Design review of the part built by this model. Coordinates are the model's own, in mm. A direction names the side the tool comes from. Coordinates: 2 decimals unless noted, no trailing zeros. Loops run counter-clockwise (first coordinate to the right, second up) from the corner with the lowest first, then second, coordinate; pieces in that order, holes last. Notation, with made-up numbers: (73, -8.5) - (104, -8.5) arc R20 ccw to (104, 0.5) - close; hole circle Ø4 at (58, -33.75). An arc over 180 degrees is marked (long way). One line per question, with ' | ' between items.
from build123d import *

# Parameters (mm, degrees)
SKETCH1_W           = 12.7
SKETCH1_H           = 12.7
BOSS_EXTRUDE1_DEPTH = 2.54
FILLET1_R           = 0.635
SHELL1_START        = 0.635
SHELL1_OUTLINE_W    = 1.905
SHELL1_OUTLINE_H    = 11.43
SHELL1_DEPTH        = 11.43
SKETCH2_R           = 2.54
BOSS_EXTRUDE2_DEPTH = 1.905
BOSS_EXTRUDE3_DEPTH = 0.00254


# Read off the part's stored shape, not the designer's step: Shell1
with BuildPart() as part:
    # Sketch1 → Boss-Extrude1 (new body)
    with BuildSketch(Plane(origin=(0, 0, 0), x_dir=(1, 0, 0), z_dir=(0, 1, 0))):
        with Locations((6.35, 6.35)):
            Rectangle(SKETCH1_W, SKETCH1_H)
    extrude(amount=BOSS_EXTRUDE1_DEPTH)

    # Fillet1
    fillet1_edges = [part.edges().sort_by_distance(p)[0] for p in [
        (0, 1.27, -12.7),
        (12.7, 1.27, -12.7),
        (12.7, 1.27, 0),
        (0, 1.27, 0),
    ]]
    fillet(fillet1_edges, radius=FILLET1_R)

    # Shell1 outline → Shell1 (cut)
    with BuildSketch(Plane.YZ.offset(SHELL1_START)):
        with Locations((0.9525, -6.35)):
            Rectangle(SHELL1_OUTLINE_W, SHELL1_OUTLINE_H)
    extrude(amount=SHELL1_DEPTH, mode=Mode.SUBTRACT)

    # Sketch2 → Boss-Extrude2 (add)
    with BuildSketch(Plane(origin=(0, 1.905, 0), x_dir=(-1, 0, 0), z_dir=(0, -1, 0))):
        with Locations(Location((-6.35, 6.35, 0), (0, 0, 270))):
            Circle(SKETCH2_R)
    extrude(amount=BOSS_EXTRUDE2_DEPTH)

    # Sketch3 → Boss-Extrude3 (add)
    with BuildSketch(Plane(origin=(0, 2.54, 0), x_dir=(1, 0, 0), z_dir=(0, 1, 0))):
        Polygon((7.227602564, 7.885397436), (7.227602564, 7.341602364), (5.070230769, 8.455269231), (5.070230769, 8.903661659), (7.227602564, 10.017328526), (7.227602564, 9.472897436), (5.689711939, 8.679147436), align=None)
        Polygon((6.310271795, 4.143044271), (6.717323077, 3.932522436), (6.198332692, 3.026833333), (5.91212476, 3.166121194), align=None)
    extrude(amount=BOSS_EXTRUDE3_DEPTH)


solid = part.part
Q1. Take a section at B-B (z = -6.35). Give the boundary of the cut face in (x, y) (3 decimals).
Returned:
outline: (0, 0) - (0.635, 0) - (0.635, 1.905) - (3.81, 1.905) - (3.81, 0) - (8.89, 0) - (8.89, 1.905) - (12.065, 1.905) - (12.065, 0) - (12.7, 0) - (12.7, 2.54) - (0, 2.54) - close
Q2. To check wall thickness, follow line 1 along X through (y, z) = (1.6, -10.25) (3 decimals); line 2 along Z through (x, y) = (7.5, 0.2) (3 decimals); line 3 along Z through (x, y) = (3.75, 1.35) (3 decimals). State the ranges of each line that lie inside material, in increasing order.
Returned:
line 1: x = 0 to 0.635, 12.065 to 12.7 | line 2: z = -12.7 to -12.065, -8.615 to -4.085, -0.635 to 0 | line 3: z = -12.7 to -12.065, -0.635 to 0
Q3. For pin 1 (3 mm diameter, centred on x = 2, z = -11, fed in from +Y), flat-tipped, find the tip position at first contact; note if it passes through.
Returned:
pin 1: stops at y = 2.54
Q4. Take a section at C-C (x = 10.75). Give the boundary of the cut face in (y, z) (3 decimals).
Returned:
outline: (0, -12.7) - (2.54, -12.7) - (2.54, 0) - (0, 0) - (0, -0.635) - (1.905, -0.635) - (1.905, -12.065) - (0, -12.065) - close
Q5. Take a section at A-A (y = 0.95). Give the boundary of the cut face in (x, z) (3 decimals).
Returned:
outline: (0, -12.065) arc R0.635 ccw to (0.635, -12.7) - (12.065, -12.7) arc R0.635 ccw to (12.7, -12.065) - (12.7, -0.635) arc R0.635 ccw to (12.065, 0) - (0.635, 0) arc R0.635 ccw to (0, -0.635) - close; circle Ø5.08 at (6.35, -6.35); hole (0.635, -12.065) - (12.065, -12.065) - (12.065, -0.635) - (0.635, -0.635) - close
Q6. Tool access review of faces 1 (the flat face through (12.065, 1, -6)), 2 (the flat face through (5.9, 2.543, -8.4)): name each direction out of +Z, -Z, +X, -X, +Y, -Y from which nothing blocks a thin tool from reaching the whole face with its end or side.
Returned:
face 1: -Y | face 2: +Z, -Z, +X, -X, +Y
Q7. Draft analysis for pull direction X (two halves, no side actions). For faces 3 (the flat face through (6, 0, -6)), 4 (the flat face through (0, 1, -6)), 5 (the flat face through (12.7, 1, -6)), 6 (the flat face through (0.635, 1, -6)), state which applies: +X half, -X half, draft (parallel to the pull), parting line (faces both ways), or undercut.
Returned:
face 3: draft | face 4: -X half | face 5: +X half | face 6: undercut
